Source: CAD feature listing. Evaluate the final solid. Frame: model axes, mm. Face numbers are marked on the shaded views. A direction names the side the tool comes from. Round coordinates to 2 decimals unless told otherwise and drop trailing zeros. Write each loop counter-clockwise with the first axis right and the second up, starting at its lowest first coordinate (ties: lowest second). Pieces come first, ordered by that corner, then holes.
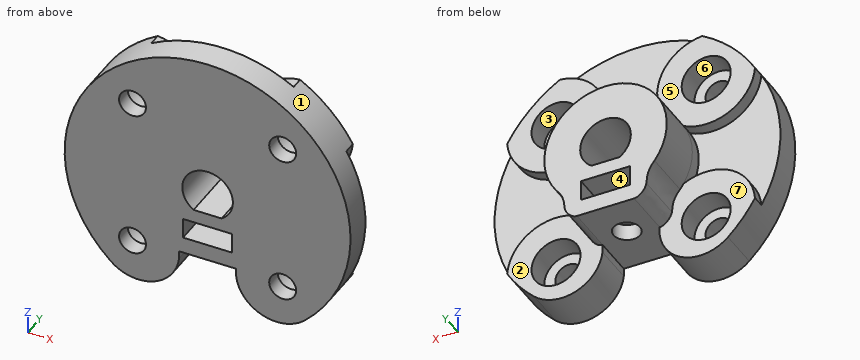
from build123d import *

# Parameters (mm, degrees)
SKETCH_1_R               = 17.5
EXTRUDE_1_DEPTH          = 2
SKETCH_2_R               = 8.75
EXTRUDE_2_DEPTH          = 9
CUT_EXTRUDE_START        = -2
CUT_EXTRUDE_8_DEPTH      = 2
SKETCH_9_R               = 1.65
CUT_EXTRUDE_7_DEPTH      = 27.334388165
PATTERN_CIRCULAR_2_COUNT = 4
SKETCH_10_R              = 17.5
SKETCH_10_R_2            = 8.75
SKETCH_10_R_3            = 3
EXTRUDE_3_DEPTH          = 3
SKETCH_14_W              = 7
SKETCH_14_H              = 5
CUT_EXTRUDE_9_DEPTH      = 34.411263071
SKETCH_3_R               = 1.625
CUT_EXTRUDE_1_DEPTH      = 29.922359862
SKETCH_4_W               = 6
SKETCH_4_H               = 2.5
CUT_EXTRUDE_2_DEPTH      = 28.083205128
SKETCH_11_R              = 1.625
EXTRUDE_4_DEPTH          = 3
FILLET_2_R               = 5
CUT_EXTRUDE_START_2      = -6
CUT_EXTRUDE_11_DEPTH     = 6
CUT_EXTRUDE_START_3      = -1.5
CUT_EXTRUDE_12_DEPTH     = 1.5
EXTRUDE_5_DEPTH          = 11
CUT_EXTRUDE_START_4      = -1
SKETCH_19_R              = 1.625
CUT_EXTRUDE_13_DEPTH     = 1
CUT_EXTRUDE_15_DEPTH     = 6


with BuildPart() as part:
    # Эскиз1 → Бобышка-Вытянуть1 (new body)
    with BuildSketch(Plane(origin=(0, 0, 0), x_dir=(1, 0, 0), z_dir=(0, 1, 0))):
        with Locations(Location((0, 0, 0), (0, 0, 270))):
            Circle(SKETCH_1_R)
    extrude(amount=EXTRUDE_1_DEPTH)

    # Эскиз2 → Бобышка-Вытянуть2 (add)
    with BuildSketch(Plane(origin=(0, 2, 0), x_dir=(1, 0, 0), z_dir=(0, 1, 0))):
        with Locations(Location((0, 0, 0), (0, 0, 270))):
            Circle(SKETCH_2_R)
        with BuildLine():
            Line((-1.763405796, 2.73), (1.763405796, 2.73))
            ThreePointArc((1.763405796, 2.73), (0, -3.25), (-1.763405796, 2.73))
        make_face(mode=Mode.SUBTRACT)
    extrude(amount=EXTRUDE_2_DEPTH)

    # Эскиз12 → Вырез-Вытянуть8 (cut)
    with BuildSketch(Plane(origin=(0, 2, 0), x_dir=(1, 0, 0), z_dir=(0, 1, 0)).offset(CUT_EXTRUDE_START)):
        with BuildLine():
            Line((-1.763405796, 2.73), (1.763405796, 2.73))
            ThreePointArc((1.763405796, 2.73), (0, -3.25), (-1.763405796, 2.73))
        make_face()
    extrude(amount=CUT_EXTRUDE_8_DEPTH, mode=Mode.SUBTRACT)

    # Эскиз9 → Вырез-Вытянуть7 (cut, through all)
    with BuildSketch(Plane(origin=(0, 2, 0), x_dir=(1, 0, 0), z_dir=(0, 1, 0))):
        with Locations(Location((9.192388155, 9.192388155, 0), (0, 0, 270))):
            Circle(SKETCH_9_R)
    cut_extrude_7 = extrude(amount=-CUT_EXTRUDE_7_DEPTH, mode=Mode.SUBTRACT)

    # Круговой массив2: Вырез-Вытянуть7 ×4 about axis
    pattern_circular_2_axis = Axis((0, 0, 0), (0, 1, 0))
    for i in range(1, PATTERN_CIRCULAR_2_COUNT):
        add(cut_extrude_7.rotate(pattern_circular_2_axis, i * 360 / PATTERN_CIRCULAR_2_COUNT), mode=Mode.SUBTRACT)

    # Эскиз10 → Бобышка-Вытянуть3 (add)
    with BuildSketch(Plane(origin=(0, 2, 0), x_dir=(1, 0, 0), z_dir=(0, 1, 0))):
        with Locations(Location((0, 0, 0), (0, 0, 270))):
            Circle(SKETCH_10_R)
        with Locations(Location((0, 0, 0), (0, 0, 270))):
            Circle(SKETCH_10_R_2, mode=Mode.SUBTRACT)
        with Locations(Location((-9.192388155, 9.192388155, 0), (0, 0, 270))):
            Circle(SKETCH_10_R_3, mode=Mode.SUBTRACT)
        with Locations(Location((9.192388155, 9.192388155, 0), (0, 0, 270))):
            Circle(SKETCH_10_R_3, mode=Mode.SUBTRACT)
        with Locations(Location((9.192388155, -9.192388155, 0), (0, 0, 270))):
            Circle(SKETCH_10_R_3, mode=Mode.SUBTRACT)
        with Locations(Location((-9.192388155, -9.192388155, 0), (0, 0, 270))):
            Circle(SKETCH_10_R_3, mode=Mode.SUBTRACT)
    extrude(amount=EXTRUDE_3_DEPTH)

    # Эскиз14 → Вырез-Вытянуть9 (cut, through all)
    with BuildSketch(Plane(origin=(0, 0, -8.75), x_dir=(-1, 0, 0), z_dir=(0, 0, -1))):
        with Locations((0, 2.5)):
            Rectangle(SKETCH_14_W, SKETCH_14_H)
    extrude(amount=CUT_EXTRUDE_9_DEPTH, mode=Mode.SUBTRACT)

    # Эскиз3 → Вырез-Вытянуть1 (cut, through all)
    with BuildSketch(Plane.XY.offset(-2.73)):
        with Locations((0, 6)):
            Circle(SKETCH_3_R)
    extrude(amount=-CUT_EXTRUDE_1_DEPTH, mode=Mode.SUBTRACT)

    # Эскиз4 → Вырез-Вытянуть2 (cut, through all)
    with BuildSketch(Plane(origin=(0, 11, 0), x_dir=(1, 0, 0), z_dir=(0, 1, 0))):
        with Locations((0, 5.48)):
            Rectangle(SKETCH_4_W, SKETCH_4_H)
    extrude(amount=-CUT_EXTRUDE_2_DEPTH, mode=Mode.SUBTRACT)

    # Эскиз11 → Бобышка-Вытянуть4 (add)
    with BuildSketch(Plane.XY.offset(-6.73)):
        Polygon((5, 1), (3.5, 1), (3.5, 0), (-3.5, 0), (-3.5, 1), (-5, 1), (-5, 11), (5, 11), align=None)
        with Locations((0, 6)):
            Circle(SKETCH_11_R, mode=Mode.SUBTRACT)
    extrude(amount=-EXTRUDE_4_DEPTH)

    # Скругление2
    # the kernel refuses this fillet: 5 mm, written as the material it takes off along each edge
    with BuildSketch(Plane(origin=(3.5, 28.475665973, -17.146428199), x_dir=(0.8902152374524571, 0, 0.4555401530133928), z_dir=(0, -1, 0))) as fillet_2_piece_1:
        with BuildLine():
            CenterArc((8.048799762, 4.816686339), FILLET_2_R, 159.077415517, 126.48531946)
            Line((3.378480837, 6.602217391), (3.285074458, 6.637928012))
            ThreePointArc((3.285074458, 6.637928012), (1.600218895, 3.346662711), (-0.089021524, 0.045554015))
            Line((-0.089021524, 0.045554015), (-0.026829333, -0.096333727))
            ThreePointArc((-0.026829333, -0.096333727), (4.695133195, -0.741597813), (9.417095722, -0.096333727))
            Line((9.417095722, -0.096333727), (9.390266389, 0))
        make_face()
    extrude(amount=51.951331945, mode=Mode.SUBTRACT)
    with BuildSketch(Plane(origin=(-3.5, 28.475665973, -17.146428199), x_dir=(-0.8902152374524572, 0, 0.4555401530133924), z_dir=(0, -1, 0))) as fillet_2_piece_2:
        with BuildLine():
            CenterArc((8.048799762, -4.816686339), FILLET_2_R, 74.437265023, 126.48531946)
            Line((3.378480837, -6.602217391), (3.285074458, -6.637928012))
            ThreePointArc((3.285074458, -6.637928012), (1.600218895, -3.346662711), (-0.089021524, -0.045554015))
            Line((-0.089021524, -0.045554015), (-0.026829333, 0.096333727))
            ThreePointArc((-0.026829333, 0.096333727), (4.695133195, 0.741597813), (9.417095722, 0.096333727))
            Line((9.417095722, 0.096333727), (9.390266389, 0))
        make_face()
    extrude(amount=51.951331945, mode=Mode.SUBTRACT)

    # Эскиз16 → Вырез-Вытянуть11 (cut)
    with BuildSketch(Plane(origin=(0, 11, 0), x_dir=(1, 0, 0), z_dir=(0, 1, 0)).offset(CUT_EXTRUDE_START_2)):
        with BuildLine():
            Line((-6, 4.5), (-5, 7.180703308))
            ThreePointArc((-5, 7.180703308), (0, -8.75), (5, 7.180703308))
            Line((5, 7.180703308), (6, 4.5))
            ThreePointArc((6, 4.5), (0, -7.5), (-6, 4.5))
        make_face()
    extrude(amount=CUT_EXTRUDE_11_DEPTH, mode=Mode.SUBTRACT)

    # Эскиз17 → Вырез-Вытянуть12 (cut)
    with BuildSketch(Plane(origin=(0, 5, 0), x_dir=(1, 0, 0), z_dir=(0, 1, 0)).offset(CUT_EXTRUDE_START_3)):
        with BuildLine():
            ThreePointArc((-15.17363778, 8.718412499), (-17.5, 0), (-15.17363778, -8.718412499))
            ThreePointArc((-15.17363778, -8.718412499), (-12.101500502, -3.944811061), (-6.425279536, -3.868563413))
            ThreePointArc((-6.425279536, -3.868563413), (-7.5, 0), (-6.425279536, 3.868563413))
            ThreePointArc((-6.425279536, 3.868563413), (-12.101500502, 3.944811061), (-15.17363778, 8.718412499))
        make_face()
        with BuildLine():
            ThreePointArc((-8.718412499, -15.17363778), (0, -17.5), (8.718412499, -15.17363778))
            ThreePointArc((8.718412499, -15.17363778), (3.944811061, -12.101500502), (3.868563413, -6.425279536))
            ThreePointArc((3.868563413, -6.425279536), (0, -7.5), (-3.868563413, -6.425279536))
            ThreePointArc((-3.868563413, -6.425279536), (-3.944811061, -12.101500502), (-8.718412499, -15.17363778))
        make_face()
        with BuildLine():
            ThreePointArc((15.17363778, -8.718412499), (17.5, 0), (15.17363778, 8.718412499))
            ThreePointArc((15.17363778, 8.718412499), (12.101500502, 3.944811061), (6.425279536, 3.868563413))
            ThreePointArc((6.425279536, 3.868563413), (7.5, 0), (6.425279536, -3.868563413))
            ThreePointArc((6.425279536, -3.868563413), (12.101500502, -3.944811061), (15.17363778, -8.718412499))
        make_face()
    extrude(amount=CUT_EXTRUDE_12_DEPTH, mode=Mode.SUBTRACT)

    # Эскиз18 → Бобышка-Вытянуть5 (add, through all)
    with BuildSketch(Plane(origin=(0, 11, 0), x_dir=(1, 0, 0), z_dir=(0, 1, 0))):
        with BuildLine():
            Line((-1.763405796, 2.73), (1.763405796, 2.73))
            ThreePointArc((1.763405796, 2.73), (0, -3.25), (-1.763405796, 2.73))
        make_face()
        with BuildLine():
            Line((-1.718604085, 2.58), (1.718604085, 2.58))
            ThreePointArc((1.718604085, 2.58), (0, -3.1), (-1.718604085, 2.58))
        make_face(mode=Mode.SUBTRACT)
    extrude(amount=-EXTRUDE_5_DEPTH)

    # Эскиз19 → Вырез-Вытянуть13 (cut)
    with BuildSketch(Plane(origin=(0, 0, -9.73), x_dir=(-1, 0, 0), z_dir=(0, 0, -1)).offset(CUT_EXTRUDE_START_4)):
        Polygon((-5, 11), (5, 11), (5, 5), (3.5, 5), (3.5, 0), (-3.5, 0), (-3.5, 5), (-5, 5), align=None)
        with Locations(Location((0, 6, 0), (0, 0, 180))):
            Circle(SKETCH_19_R, mode=Mode.SUBTRACT)
    extrude(amount=CUT_EXTRUDE_13_DEPTH, mode=Mode.SUBTRACT)

    # Эскиз20 → Вырез-Вытянуть15 (cut)
    with BuildSketch(Plane(origin=(0, 11, 0), x_dir=(1, 0, 0), z_dir=(0, 1, 0))):
        with BuildLine():
            add(Edge.make_bspline(
                [(-3.5, 8.73), (-4.079656123, 8.73), (-4.842651299, 7.966190202), (-4.988696176, 7.252329412), (-5, 7.180703308)],
                knots=[0, 0, 0, 0, 0.430033256, 0.477814729, 0.477814729, 0.477814729, 0.477814729], degree=3))
            Line((-3.5, 8.73), (-5, 8.73))
            Line((-5, 8.73), (-5, 7.180703308))
        make_face()
        with BuildLine():
            add(Edge.make_bspline(
                [(-5, 7.180703308), (-5.012353513, 7.102425904), (-5.096467294, 6.31678513), (-5.16082419, 5.405951438), (-6, 4.5)],
                knots=[0.477814729, 0.477814729, 0.477814729, 0.477814729, 0.530033256, 1, 1, 1, 1], degree=3))
            Line((-5, 7.180703308), (-6, 4.5))
        make_face()
        with BuildLine():
            Line((5, 8.73), (3.5, 8.73))
            add(Edge.make_bspline(
                [(3.5, 8.73), (4.079656123, 8.73), (4.842651299, 7.966190202), (4.988696176, 7.252329412), (5, 7.180703308)],
                knots=[0, 0, 0, 0, 0.430033256, 0.477814729, 0.477814729, 0.477814729, 0.477814729], degree=3))
            Line((5, 7.180703308), (5, 8.73))
        make_face()
        with BuildLine():
            Line((6, 4.5), (5, 7.180703308))
            add(Edge.make_bspline(
                [(5, 7.180703308), (5.012353513, 7.102425904), (5.096467294, 6.31678513), (5.16082419, 5.405951438), (6, 4.5)],
                knots=[0.477814729, 0.477814729, 0.477814729, 0.477814729, 0.530033256, 1, 1, 1, 1], degree=3))
        make_face()
    extrude(amount=-CUT_EXTRUDE_15_DEPTH, mode=Mode.SUBTRACT)


solid = part.part
1) Section query C-C on y = 1.25. Return the cut outline in (x, z), then the cut area to 3 significant figures.
Taken from the geometry:
outline: (-11.86, -12.87) arc R5 ccw to (-3.5, -9.73) - (-3.5, -8.73) - (3.5, -8.73) - (3.5, -9.73) arc R5 ccw to (11.86, -12.87) arc R17.5 ccw (long way) to start; hole circle Ø3.3 at (-9.19, -9.19); hole circle Ø3.3 at (-9.19, 9.19); hole (-3, -6.73) - (3, -6.73) - (3, -4.23) - (-3, -4.23) - close; hole (-1.72, -2.58) - (1.72, -2.58) arc R3.1 ccw (long way) to start; hole circle Ø3.3 at (9.19, -9.19); hole circle Ø3.3 at (9.19, 9.19)
area: 788 mm2
2) Material intervals for line 1 (Z direction, x = 0, y = 7.25); line 2 (X direction, y = 2.5, z = 0); line 3 (X direction, y = 2.75, z = -11), sorted ascending.
Taken from the geometry:
line 1: z = -2.73 to -2.58, 3.1 to 7.5
line 2: x = -17.5 to -3.1, 3.1 to 17.5
line 3: x = -13.61 to -11.59, -6.8 to -3.81, 3.81 to 6.8, 11.59 to 13.61
3) Section query A-A on x = 0. Return the cut outline in (y, z) (3 decimals), then the cut area to 3 significant figures.
Taken from the geometry:
outline: (0, -8.73) - (4.375, -8.73) - (4.375, -6.73) - (0, -6.73) - close; (0, -4.23) - (4.375, -4.23) - (4.375, -2.73) - (7.625, -2.73) - (7.625, -4.23) - (11, -4.23) - (11, -2.58) - (0, -2.58) - close; (0, 3.1) - (11, 3.1) - (11, 7.5) - (3.5, 7.5) - (3.5, 17.5) - (0, 17.5) - close; (7.625, -8.73) - (11, -8.73) - (11, -6.73) - (7.625, -6.73) - close
area: 112 mm2
4) Section query D-D on z = 10. Return the cut outline in (x, y).
Taken from the geometry:
outline: (-14.36, 0) - (-10.63, 0) - (-10.63, 2) - (-12.08, 2) - (-12.08, 5) - (-14.36, 5) - close; (-7.75, 0) - (7.75, 0) - (7.75, 2) - (6.3, 2) - (6.3, 5) - (3.25, 5) - (3.25, 3.5) - (-3.25, 3.5) - (-3.25, 5) - (-6.3, 5) - (-6.3, 2) - (-7.75, 2) - close; (10.63, 0) - (14.36, 0) - (14.36, 5) - (12.08, 5) - (12.08, 2) - (10.63, 2) - close
5) Pull-direction query (Z, two-part tool) for the marked faces 1, 2 and 3; classes: released by +Z, released by -Z, zero draft, split by the parting line, or undercut.
Taken from the geometry:
face 1: split by the parting line
face 2: zero draft
face 3: undercut
6) Section query B-B on z = 0. Return the cut outline in (x, y), then the cut area to 3 significant figures.
Taken from the geometry:
outline: (-17.5, 0) - (-3.1, 0) - (-3.1, 11) - (-7.5, 11) - (-7.5, 3.5) - (-17.5, 3.5) - close; (3.1, 0) - (17.5, 0) - (17.5, 3.5) - (7.5, 3.5) - (7.5, 11) - (3.1, 11) - close
area: 167 mm2
7) Reachability of the marked faces 4, 5, 6 and 7 from +Z, -Z, +X, -X, +Y, -Y: full face, straight path, thin tool, end or side. Return the list, or none.
Taken from the geometry:
face 4: +Y, -Y
face 5: +Z, -X, +Y
face 6: +Y
face 7: -Z, -X, +Y
8) Contact query for flat-ended pins moving along their axis: P1, Ø13, axis at x = 12, z = 8.5, coming from the +Y side; P2, Ø2, axis at y = 5, z = 0.5, coming from the -X side; P3, Ø0.5, axis at y = 2, z = -9.5, coming from the -X side. Output: stop coordinate, or through.
Taken from the geometry:
P1: stops at y = 5
P2: stops at x = -7.5
P3: stops at x = -14.86
